Geometry check sheet. Reference: the model listing, model coordinates, mm. A direction names the side the tool comes from. Coordinates: 2 decimals unless noted, no trailing zeros. Write each loop counter-clockwise with the first axis right and the second up, starting at its lowest first coordinate (ties: lowest second). Pieces come first, ordered by that corner, then holes. Notation, with made-up numbers: (-34.5, -33) -> (-17.5, -33) arc R9 cw to (-17.5, -19) -> close; hole circle Ø4 at (41.25, 82). An arc over 180 degrees is marked (long way). Put each result on its own line as item: value. Start each with the question number.
from build123d import *

# Parameters (mm, degrees)
BOSS_EXTRU_1_DEPTH      = 97
ESQUISSE2_W             = 12
ESQUISSE2_H             = 5
ENL_V_MAT_EXTRU_1_DEPTH = 10


with BuildPart() as part:
    # Esquisse1 → Boss.-Extru.1 (new body)
    with BuildSketch(Plane.XY):
        with BuildLine():
            Line((0, 11), (58, 11))
            ThreePointArc((58, 11), (69, 0), (58, -11))
            Line((58, -11), (0, -11))
            ThreePointArc((0, -11), (-11, 0), (0, 11))
        make_face()
    extrude(amount=BOSS_EXTRU_1_DEPTH)

    # Esquisse2 → Enlèv. mat.-Extru.1 (cut)
    with BuildSketch(Plane.XY.offset(97)):
        with BuildLine():
            Line((0, -1), (7, -1))
            ThreePointArc((7, -1), (8, -2), (7, -3))
            Line((7, -3), (0, -3))
            ThreePointArc((0, -3), (-1, -2), (0, -1))
        make_face()
        with Locations((52, 0)):
            Rectangle(ESQUISSE2_W, ESQUISSE2_H)
        with Locations((34, 0)):
            Rectangle(ESQUISSE2_W, ESQUISSE2_H)
    extrude(amount=-ENL_V_MAT_EXTRU_1_DEPTH, mode=Mode.SUBTRACT)


solid = part.part
Item 1: Section check D-D, the plane x = -4. Enter the section's corners in (y, z), and give its area (3 significant figures).
Item 2: Go/stop test with a flat-tipped pin: P1, Ø12, axis at y = -7, z = 33.5, coming from the +X side. Record where the tip stops, or that it passes through.
Item 3: Section check B-B, the plane y = 0.75. Enter the section's corners in (x, z).
Item 4: Section check C-C, the plane z = 30. Enter the section's corners in (x, y), and give its area (3 significant figures).
Item 5: Section check A-A, the plane x = 31. Enter the section's corners in (y, z), and give its area (3 significant figures).
Item 6: Access from +Z, -Z, +X, -X, +Y, -Y to the whole of each face (thin tool, end or side, straight path). Record for faces 1 (the flat face through (4, -3, 92)), 2 (the flat face through (29, 11, 48)).
Item 7: Scan lines: line 1 along X through (y, z) = (-0.25, 32.5); line 2 along Z through (x, y) = (49, 0.75); line 3 along Y through (x, z) = (-7, 22.5). Record each from-to range of solid material in increasing order. Write a range as [from, to].
Item 8: Mould release check, pull along X, two halves, no side actions. Record for faces 3 (the cylindrical face through (69, 0, 48)), 4 (the cylindrical face through (-1, -2, 92)), 5 (the cylindrical face through (-11, 0, 48)), 6 (the flat face through (30, 3, 97)): released by +X, released by -X, zero draft, split by the parting line, or undercut.
From the geometry:
1. outline: (-10.25, 0) -> (10.25, 0) -> (10.25, 97) -> (-10.25, 97) -> close
1. area: 1,990 mm²
2. P1: x = 68.95
3. outline: (-10.97, 0) -> (68.97, 0) -> (68.97, 97) -> (58, 97) -> (58, 87) -> (46, 87) -> (46, 97) -> (40, 97) -> (40, 87) -> (28, 87) -> (28, 97) -> (-10.97, 97) -> close
4. outline: (0, -11) -> (58, -11) arc R11 ccw to (58, 11) -> (0, 11) arc R11 ccw to start
4. area: 1,660 mm²
5. outline: (-11, 0) -> (11, 0) -> (11, 97) -> (2.5, 97) -> (2.5, 87) -> (-2.5, 87) -> (-2.5, 97) -> (-11, 97) -> close
5. area: 2,080 mm²
6. face 1: +Z
6. face 2: +Z, -Z, +X, -X, +Y
7. line 1: [-11, 69]
7. line 2: [0, 87]
7. line 3: [-8.49, 8.49]
8. face 3: released by +X
8. face 4: undercut
8. face 5: released by -X
8. face 6: zero draft
